Build history of the part. All positions in model axes, mm. Face numbers are marked on the shaded views. A direction names the side the tool comes from. Give positions to 0.01 mm unless a question says otherwise; leave off trailing zeros. Write each loop counter-clockwise with the first axis right and the second up, starting at its lowest first coordinate (ties: lowest second). Pieces come first, ordered by that corner, then holes. Notation, with made-up numbers: M 21,45.5 L 76,45.5 A13 ccw 76,52.5 Z; hole C 8.5,40.25 d5. An arc over 180 degrees is marked long. One line per item, written item: value. Start each with the question number.
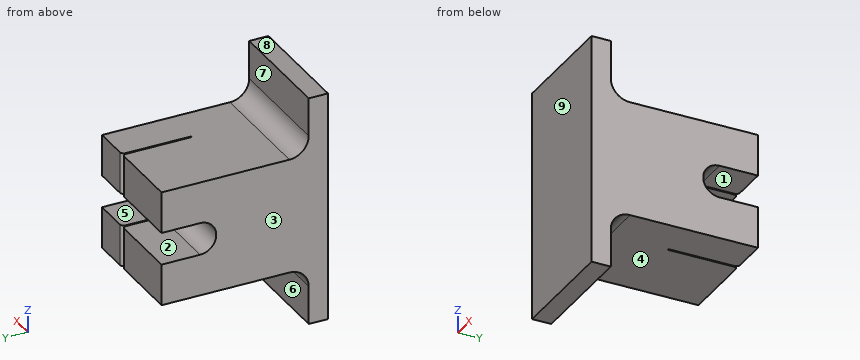
from build123d import *

# Parameters (mm, degrees)
SKETCH1_W           = 30
SKETCH1_H           = 30
BOSS_EXTRUDE1_DEPTH = 33.2
SKETCH2_R           = 4.205
CUT_EXTRUDE1_DEPTH  = 48.19364364
SKETCH4_W           = 60
SKETCH4_H           = 5
BOSS_EXTRUDE2_DEPTH = 30
FILLET1_R           = 5
SKETCH5_W           = 30
SKETCH5_H           = 10.795
BOSS_EXTRUDE3_DEPTH = 10
SKETCH6_W           = 0.33
SKETCH6_H           = 30
CUT_EXTRUDE2_DEPTH  = 18
FILLET2_R           = 1


with BuildPart() as part:
    # Sketch1 → Boss-Extrude1 (new body)
    with BuildSketch(Plane(origin=(0, 0, 0), x_dir=(1, 0, 0), z_dir=(0, 1, 0))):
        Rectangle(SKETCH1_W, SKETCH1_H)
    extrude(amount=BOSS_EXTRUDE1_DEPTH)

    # Sketch2 → Cut-Extrude1 (cut, through all)
    with BuildSketch(Plane.ZY.offset(15)):
        with Locations((0, 33.2)):
            Circle(SKETCH2_R)
    extrude(amount=-CUT_EXTRUDE1_DEPTH, mode=Mode.SUBTRACT)

    # Sketch4 → Boss-Extrude2 (add)
    with BuildSketch(Plane(origin=(15, 0, 0), x_dir=(0, 0, -1), z_dir=(1, 0, 0))):
        with Locations((0, 2.5)):
            Rectangle(SKETCH4_W, SKETCH4_H)
    extrude(amount=-BOSS_EXTRUDE2_DEPTH)

    # Fillet1
    fillet1_edges = [part.edges().sort_by_distance(p)[0] for p in [
        (0, 5, -15),
        (0, 5, 15),
    ]]
    fillet(fillet1_edges, radius=FILLET1_R)

    # Sketch5 → Boss-Extrude3 (add)
    with BuildSketch(Plane(origin=(0, 33.2, 0), x_dir=(1, 0, 0), z_dir=(0, 1, 0))):
        with Locations((0, 9.6025)):
            Rectangle(SKETCH5_W, SKETCH5_H)
        with Locations((0, -9.6025)):
            Rectangle(SKETCH5_W, SKETCH5_H)
    extrude(amount=BOSS_EXTRUDE3_DEPTH)

    # Sketch6 → Cut-Extrude2 (cut)
    with BuildSketch(Plane(origin=(0, 43.2, 0), x_dir=(1, 0, 0), z_dir=(0, 1, 0))):
        with Locations((4.835, 0)):
            Rectangle(SKETCH6_W, SKETCH6_H)
    extrude(amount=-CUT_EXTRUDE2_DEPTH, mode=Mode.SUBTRACT)

    # Fillet2
    fillet2_edges = [part.edges().sort_by_distance(p)[0] for p in [
        (5, 43.2, -9.6025),
        (5, 43.2, 9.6025),
        (4.67, 43.2, 9.6025),
        (4.67, 43.2, -9.6025),
    ]]
    fillet(fillet2_edges, radius=FILLET2_R)


solid = part.part
1) Band-saw the part on D-D (z = 0). List the corners of the cut face in (x, y) (3 decimals), then the cut area to 3 significant figures.
2) Band-saw the part on A-A (y = 35). List the corners of the cut face in (x, z) (3 decimals).
3) Band-saw the part on B-B (y = 26). List the corners of the cut face in (x, z).
4) Drop flat-ended pins along their axis: P1, Ø3, axis at x = 2, y = 8, coming from the +Z side; P2, Ø5, axis at x = -7, z = -24.5, coming from the +Y side; P3, Ø5, axis at x = -8.5, y = 36, coming from the -Z side. Give the stop position or say it passes through.
5) Band-saw the part on C-C (x = -11.75). List the corners of the cut face in (y, z) (3 decimals), then the cut area to 3 significant figures.
6) Mould opens along Z. For the marked faces 1, 2, 3 and 4 say: released by +Z, released by -Z, zero draft, split by the parting line, or undercut.
7) Tool access for the marked faces 5, 6, 7, 8 and 9: list every direction of +Z, -Z, +X, -X, +Y, -Y with a clear straight run to the whole face (end or side of a thin tool).
8) Probe line 1 along Z through (x, y) = (8.25, 38) (3 decimals); line 2 along X through (y, z) = (39, -8); line 3 along Z through (x, y) = (-2.75, 19). List the from-to ranges inside material, lowest first. Write a range as from..to.
Model answer:
1. outline: M -15,0 L 15,0 L 15,28.995 L 5,28.995 L 5,25.2 L 4.67,25.2 L 4.67,28.995 L -15,28.995 Z
1. area: 869 mm²
2. outline: M -15,-15 L 4.67,-15 L 4.67,-4.205 L -15,-4.205 Z; M -15,4.205 L 4.67,4.205 L 4.67,15 L -15,15 Z; M 5,-15 L 15,-15 L 15,-4.205 L 5,-4.205 Z; M 5,4.205 L 15,4.205 L 15,15 L 5,15 Z
3. outline: M -15,-15 L 4.67,-15 L 4.67,15 L -15,15 Z; M 5,-15 L 15,-15 L 15,15 L 5,15 Z
4. P1: stops at z = 16.43
4. P2: stops at y = 5
4. P3: stops at z = -15
5. outline: M 0,-30 L 5,-30 L 5,-20 A5 cw 10,-15 L 43.2,-15 L 43.2,-4.205 L 33.2,-4.205 A4.205 cw 33.2,4.205 L 43.2,4.205 L 43.2,15 L 10,15 A5 cw 5,20 L 5,30 L 0,30 Z
5. area: 1,340 mm²
6. face 1: undercut
6. face 2: undercut
6. face 3: zero draft
6. face 4: released by -Z
7. face 5: +X, -X, +Y
7. face 6: -Z, +X, -X, +Y
7. face 7: +Z, +X, -X, +Y
7. face 8: +Z, +X, -X, +Y, -Y
7. face 9: +Z, -Z, +X, -X, -Y
8. line 1: z = -15..-4.205, 4.205..15
8. line 2: x = -15..4.67, 5..15
8. line 3: z = -15..15
